Source: CAD feature listing. Evaluate the final solid. Frame: model axes, mm. A direction names the side the tool comes from. Coordinates: 2 decimals unless noted, no trailing zeros. Loops run counter-clockwise (first coordinate to the right, second up) from the corner with the lowest first, then second, coordinate; pieces in that order, holes last.
Item 1: Section query A-A, the plane y = -5.5. Return the cut outline in (x, z).
Item 2: Line query: probe 1 along Z at (x, y) = (17.75, -10); probe 2 along Y at (x, z) = (6.75, -20.5). Output: solid intervals per line, ascending.
Item 3: Section query D-D, the plane z = -39. Return the cut outline in (x, y).
Item 4: Section query B-B, the plane x = 12.5. Return the cut outline in (y, z).
Item 5: Pull-direction query (X, two-part tool) for faces 3 (the cylindrical face through (10.06, -13.28, 1.72)), 4 (the cylindrical face through (12.225, -25.234, -61.751)), 5 (the flat face through (10, -14, 2.737)), 6 (the cylindrical face through (10.06, -13.28, -61.75)); classes: +X half, -X half, draft (parallel to the pull), parting line (faces both ways), or undercut.
Item 6: Reachability of faces 1 (the flat face through (12, -2, -30)), 2 (the flat face through (0, -1, -30)) from +Z, -Z, +X, -X, +Y, -Y: full face, straight path, thin tool, end or side. Return the list, or none.
Item 7: Pin query (flat end, axial travel): pin 1 Ø8 at (x, z) = (18.5, -49) entering from -Y. Return the tip coordinate at first contact, or that it passes through.
Item 8: Section query C-C, the plane x = 19.75. Return the cut outline in (y, z), then the cut area to 3 significant figures.
```python
from build123d import *

# Parameters (mm, degrees)
SKETCH1_W               = 25
SKETCH1_H               = 60
BASE_FLANGE1_DEPTH      = 2
EDGE_FLANGE1_DEPTH      = 25
EDGE_FLANGE1_BEND_DEPTH = 25
CUT_EXTRUDE1_REACH      = 78.235
SKETCH12_R              = 2.5


# Sheet-metal steps are written as plain solids
with BuildPart() as part:
    # Sketch1 → Base-Flange1 (new body)
    with BuildSketch(Plane(origin=(0, 0, 0), x_dir=(1, 0, 0), z_dir=(0, 1, 0))):
        with Locations((12.5, 30)):
            Rectangle(SKETCH1_W, SKETCH1_H)
    extrude(amount=-BASE_FLANGE1_DEPTH)

    # Edge-Flange1 section (across the edge) → Edge-Flange1 (add)
    with BuildSketch(Plane(origin=(25, -2, 0.7366), x_dir=(0, 0, -1), z_dir=(-1, 0, 0))):
        with BuildLine():
            Line((-2, 0.7366), (-2, 28))
            Line((-2, 28), (0, 28))
            Line((0, 28), (0, 0.7366))
            ThreePointArc((0, 0.7366), (0.215745145, 0.215745145), (0.7366, 0))
            Line((0.7366, 0), (0.7366, -2))
            ThreePointArc((0.7366, -2), (-1.198468417, -1.198468417), (-2, 0.7366))
        make_face()
    extrude(amount=EDGE_FLANGE1_DEPTH)

    # Edge-Flange1 section 2 (across the edge) → Edge-Flange1 bend (add)
    with BuildSketch(Plane(origin=(0, -2, -60.7366), x_dir=(0, 0, 1), z_dir=(1, 0, 0))):
        with BuildLine():
            Line((-2, 0.7366), (-2, 28))
            Line((-2, 28), (0, 28))
            Line((0, 28), (0, 0.7366))
            ThreePointArc((0, 0.7366), (0.215745145, 0.215745145), (0.7366, 0))
            Line((0.7366, 0), (0.7366, -2))
            ThreePointArc((0.7366, -2), (-1.198468417, -1.198468417), (-2, 0.7366))
        make_face()
    extrude(amount=EDGE_FLANGE1_BEND_DEPTH)

    # Cut-Extrude1: up to this face of the body (flat: up to its plane)
    cut_extrude1_end = Plane(part.part.faces().sort_by_distance((12.5, -16.3683, 2.7366))[0])
    # Sketch12 → Cut-Extrude1 (cut, up to the picked face)
    with BuildSketch(Plane(origin=(0, 0, -62.7366), x_dir=(-1, 0, 0), z_dir=(0, 0, -1)), mode=Mode.PRIVATE) as cut_extrude1_sk1:
        with Locations(Location((-12.5, -12.7366, 0), (0, 0, 90))):
            Circle(SKETCH12_R)
    cut_extrude1_tool1 = split(extrude(cut_extrude1_sk1.sketch, amount=-CUT_EXTRUDE1_REACH, mode=Mode.PRIVATE), bisect_by=cut_extrude1_end, keep=Keep.BOTH, mode=Mode.PRIVATE)
    # Sketch12 → Cut-Extrude1 (cut, up to the picked face)
    with BuildSketch(Plane(origin=(0, 0, -62.7366), x_dir=(-1, 0, 0), z_dir=(0, 0, -1)), mode=Mode.PRIVATE) as cut_extrude1_sk2:
        with BuildLine():
            Line((-25, -12.7366), (-25, -30))
            Line((-25, -30), (0, -30))
            Line((0, -30), (0, -12.7366))
            ThreePointArc((0, -12.7366), (-12.5, -25.2366), (-25, -12.7366))
        make_face()
    cut_extrude1_tool2 = split(extrude(cut_extrude1_sk2.sketch, amount=-CUT_EXTRUDE1_REACH, mode=Mode.PRIVATE), bisect_by=cut_extrude1_end, keep=Keep.BOTH, mode=Mode.PRIVATE)
    add(cut_extrude1_tool1.solids().sort_by(Axis((12.5, -12.7366, -62.7366), (0, 0, 1)))[0], mode=Mode.SUBTRACT)
    add(cut_extrude1_tool2.solids().sort_by(Axis((12.5, -25.754349, -62.7366), (0, 0, 1)))[0], mode=Mode.SUBTRACT)


solid = part.part
```
Verdict:
1. outline: (0, -62.74) - (25, -62.74) - (25, -60.74) - (0, -60.74) - close; (0, 0.74) - (25, 0.74) - (25, 2.74) - (0, 2.74) - close
2. probe 1: z = -62.74 to -60.74, 0.74 to 2.74
2. probe 2: y = -2 to 0
3. outline: (0, -2) - (25, -2) - (25, 0) - (0, 0) - close
4. outline: (-25.24, -62.74) - (-15.24, -62.74) - (-15.24, -60.74) - (-25.24, -60.74) - close; (-25.24, 0.74) - (-15.24, 0.74) - (-15.24, 2.74) - (-25.24, 2.74) - close; (-10.24, -62.74) - (-2.74, -62.74) arc R2.74 ccw to (0, -60) - (0, 0) arc R2.74 ccw to (-2.74, 2.74) - (-10.24, 2.74) - (-10.24, 0.74) - (-2.74, 0.74) arc R0.74 cw to (-2, 0) - (-2, -60) arc R0.74 cw to (-2.74, -60.74) - (-10.24, -60.74) - close
5. face 3: undercut
5. face 4: parting line
5. face 5: draft
5. face 6: undercut
6. face 1: +X, -X, -Y
6. face 2: +Z, -Z, -X, +Y, -Y
7. pin 1: stops at y = -2
8. outline: (-22.92, -62.74) - (-2.74, -62.74) arc R2.74 ccw to (0, -60) - (0, 0) arc R2.74 ccw to (-2.74, 2.74) - (-22.92, 2.74) - (-22.92, 0.74) - (-2.74, 0.74) arc R0.74 cw to (-2, 0) - (-2, -60) arc R0.74 cw to (-2.74, -60.74) - (-22.92, -60.74) - close
8. area: 212 mm2
